For this review, take the finished solid that the model builds, in its own axes (mm). Face numbers are marked on the shaded views. A direction names the side the tool comes from. Round coordinates to 2 decimals unless told otherwise and drop trailing zeros. Loops run counter-clockwise (first coordinate to the right, second up) from the corner with the lowest first, then second, coordinate; pieces in that order, holes last. Notation, with made-up numbers: (87, 89.5) -> (131, 89.5) arc R31 cw to (131, 117.5) -> close; hole circle Ø2 at (75.5, 64.5). An arc over 180 degrees is marked (long way). One line per question, with ' | ' between items. Start each with the question number.
1. For pin 1 Ø3 at (x, y) = (31, 4.5) entering from +Z; pin 2 Ø12 at (x, z) = (55.5, -32.5) entering from -Y; pin 3 Ø1 at (x, y) = (-26, 6.5) entering from -Z; pin 4 Ø2 at (x, y) = (34, 6.5) entering from +Z, all flat-tipped, find the tip position at first contact; note any pin that passes through.
2. Consider section A-A (x = 0). Write out the cut boundary in (y, z), and give its area (3 significant figures).
3. Consider section D-D (z = 68.3). Write out the cut boundary in (x, y).
4. Consider section C-C (y = 3.5). Write out the cut boundary in (x, z), and give its area (3 significant figures).
5. Consider section B-B (z = 0). Write out the cut boundary in (x, y).
6. Wall thickness on line 1 along X through (y, z) = (0.75, 68.3); line 2 along X through (y, z) = (3.75, 0); line 3 along X through (y, z) = (2.5, -23.5): over which ranges is each line inside the solid? List them lowest first.
7. For the marked faces 1 and 2, list the 3-axis set-ups (+Z, -Z, +X, -X, +Y, -Y) from which the entire face can be reached by the end or side of a thin tool; tool diameter is ignored.
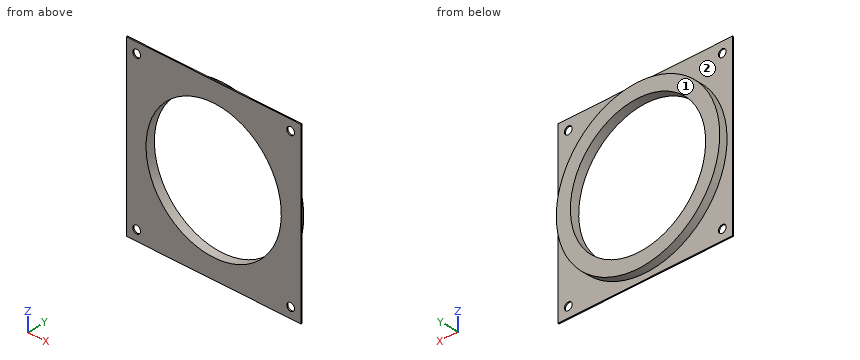
```python
from build123d import *

# Parameters (mm, degrees)
SKETCH1_W           = 155
SKETCH1_H           = 155
SKETCH1_R           = 60
SKETCH1_R_2         = 3.4
BOSS_EXTRUDE1_DEPTH = 1
SKETCH2_R           = 72.5
SKETCH2_R_2         = 60
BOSS_EXTRUDE2_DEPTH = 7


with BuildPart() as part:
    # Sketch1 → Boss-Extrude1 (new body)
    with BuildSketch(Plane(origin=(0, 0, 0), x_dir=(1, 0, 0), z_dir=(0, 1, 0))):
        Rectangle(SKETCH1_W, SKETCH1_H)
        with Locations(Location((0, 0, 0), (0, 0, 270))):
            Circle(SKETCH1_R, mode=Mode.SUBTRACT)
        with Locations(Location((-68.3, 68.3, 0), (0, 0, 270))):
            Circle(SKETCH1_R_2, mode=Mode.SUBTRACT)
        with Locations(Location((68.3, 68.3, 0), (0, 0, 90))):
            Circle(SKETCH1_R_2, mode=Mode.SUBTRACT)
        with Locations(Location((-68.3, -68.3, 0), (0, 0, 90))):
            Circle(SKETCH1_R_2, mode=Mode.SUBTRACT)
        with Locations(Location((68.3, -68.3, 0), (0, 0, 270))):
            Circle(SKETCH1_R_2, mode=Mode.SUBTRACT)
    extrude(amount=BOSS_EXTRUDE1_DEPTH)

    # Sketch2 → Boss-Extrude2 (add)
    with BuildSketch(Plane(origin=(0, 1, 0), x_dir=(1, 0, 0), z_dir=(0, 1, 0))):
        with Locations(Location((0, 0, 0), (0, 0, 270))):
            Circle(SKETCH2_R)
        with Locations(Location((0, 0, 0), (0, 0, 270))):
            Circle(SKETCH2_R_2, mode=Mode.SUBTRACT)
    extrude(amount=BOSS_EXTRUDE2_DEPTH)


solid = part.part
```
Answer block:
1) pin 1: stops at z = 66.23 | pin 2: stops at y = 0 | pin 3: stops at z = -67.87 | pin 4: stops at z = 64.55
2) outline: (0, -77.5) -> (1, -77.5) -> (1, -72.5) -> (8, -72.5) -> (8, -60) -> (0, -60) -> close; (0, 60) -> (8, 60) -> (8, 72.5) -> (1, 72.5) -> (1, 77.5) -> (0, 77.5) -> close | area: 210 mm2
3) outline: (-77.5, 0) -> (-71.7, 0) -> (-71.7, 1) -> (-77.5, 1) -> close; (-64.9, 0) -> (64.9, 0) -> (64.9, 1) -> (24.32, 1) -> (24.32, 8) -> (-24.32, 8) -> (-24.32, 1) -> (-64.9, 1) -> close; (71.7, 0) -> (77.5, 0) -> (77.5, 1) -> (71.7, 1) -> close
4) outline: circle Ø145 at (0, 0); hole circle Ø120 at (0, 0) | area: 5,200 mm2
5) outline: (-77.5, 0) -> (-60, 0) -> (-60, 8) -> (-72.5, 8) -> (-72.5, 1) -> (-77.5, 1) -> close; (60, 0) -> (77.5, 0) -> (77.5, 1) -> (72.5, 1) -> (72.5, 8) -> (60, 8) -> close
6) line 1: x = -77.5 to -71.7, -64.9 to 64.9, 71.7 to 77.5 | line 2: x = -72.5 to -60, 60 to 72.5 | line 3: x = -68.59 to -55.21, 55.21 to 68.59
7) face 1: +Z, -Z, +X, -X, +Y | face 2: +Y
